Study the drawing (mm; zero at the part's minimum x, y, z) and answer. Give positions to 0.01 mm unless a question says otherwise; leave off trailing zeros. Write each loop counter-clockwise with the first axis right and the second up, starting at its lowest first coordinate (ties: lowest second). Pieces come first, ordered by that corner, then holes.
1) Find section B-B (x = 4.25). Determine the outline of the cut face in (y, z).
2) Find section D-D (z = 31). Determine the outline of the cut face in (x, y).
3) Straight lines are drawn through the part: probe 1 along Z at (x, y) = (10.5, 6.25); probe 2 along Z at (x, y) = (14.25, 7); probe 3 along X at (y, z) = (10, 18). For each, find the intervals that lie inside material, in ascending order.
4) Find section A-A (x = 7.5). Determine the outline of the cut face in (y, z).
5) Determine the mould class of the marked faces 1, 2 and 3 for opening direction Z: pulls with the +Z half, pulls with the -Z half, needs draft (parallel to the pull), parting line crosses it, or undercut.
6) Given pin 1 Ø1 at (y, z) = (4.5, 24.5) entering from -X; pin 2 Ø1.5 at (x, z) = (5.5, 18.5) entering from +Y; pin 3 Ø8 at (x, z) = (13, 13) entering from +Y, each flat-ended and moving along its own axis, determine where each tip first touches the part or whether it passes through.
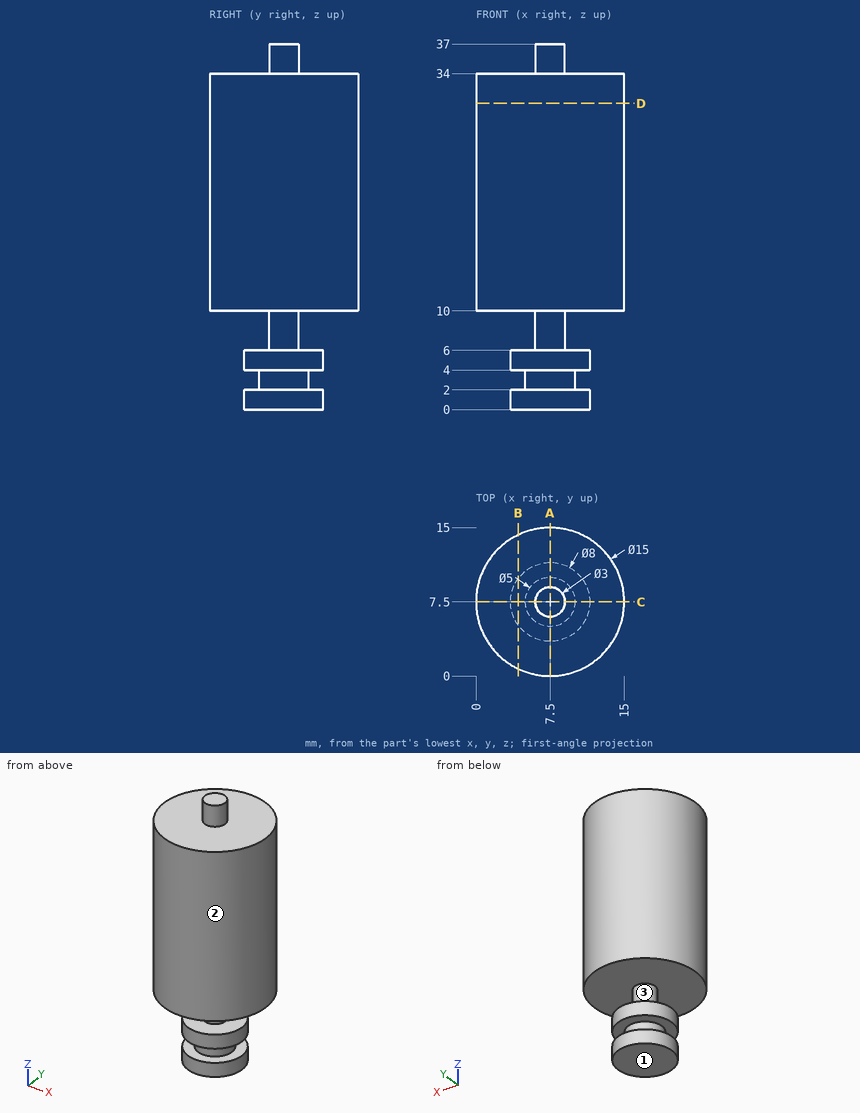
Results:
1. outline: (0.74, 10) - (14.26, 10) - (14.26, 34) - (0.74, 34) - close; (5.17, 0) - (9.83, 0) - (9.83, 2) - (5.17, 2) - close; (5.17, 4) - (9.83, 4) - (9.83, 6) - (5.17, 6) - close
2. outline: circle Ø15 at (7.5, 7.5)
3. probe 1: z = 0 to 2, 4 to 6, 10 to 34
3. probe 2: z = 10 to 34
3. probe 3: x = 0.43 to 14.57
4. outline: (0, 10) - (6, 10) - (6, 6) - (3.5, 6) - (3.5, 4) - (5, 4) - (5, 2) - (3.5, 2) - (3.5, 0) - (11.5, 0) - (11.5, 2) - (10, 2) - (10, 4) - (11.5, 4) - (11.5, 6) - (9, 6) - (9, 10) - (15, 10) - (15, 34) - (9, 34) - (9, 37) - (6, 37) - (6, 34) - (0, 34) - close
5. face 1: pulls with the -Z half
5. face 2: needs draft
5. face 3: undercut
6. pin 1: stops at x = 0.43
6. pin 2: stops at y = 14.9
6. pin 3: stops at y = 14.85
